Part model, mm, in its own coordinate system. A direction names the side the tool comes from. Give positions to 0.01 mm unless a question says otherwise; leave off trailing zeros. Order: outer loops, then holes, each group sorted by start corner. A loop starts at its lowest first (then second) coordinate and runs counter-clockwise, first axis right, second up. Notation, with made-up numbers: M -19.75,-22.75 L 13.25,-22.75 A23 ccw 13.25,-9.75 Z; hole C 24.25,48 d5. An arc over 180 degrees is marked long. Return JSON: item names as keys, results as strings.
Autodesk Inventor part; units mm, degrees
ref_plane "YZ Plane" through (0, 0, 0) normal (1, 0, 0) x (0, 1, 0)
ref_plane "XZ Plane" through (0, 0, 0) normal (0, 1, 0) x (-1, 0, 0)
ref_plane "XY Plane" through (0, 0, 0) normal (0, 0, 1) x (1, 0, 0)
sketch "Sketch1" plane through (0, 0, 0) normal (0, 1, 0) x (-1, 0, 0)
  line L0 (0, 0) -> (50.8, 0)
  line L1 (50.8, 0) -> (50.8, -9.525)
  line L2 (0, -9.525) -> (0, 0)
  line L3 (50.8, -9.525) -> (9.4322, -9.525)
  line L4 (3.3434, -9.525) -> (0, -9.525)
  arc A0 (9.4322, -9.525) -> (3.3434, -9.525) centre (6.3878, -11.9396) ccw
  point P0 (3.3434, 0)
  dimension "d1" = 9.525
revolve "Revolution1" add sketch "Sketch1" angle 360 about axis through (0, 0, 0) along (-1, 0, 0)
sketch "Sketch2" plane through (0, 0, 0) normal (1, 0, 0) x (0, 0, -1)
  circle A0 centre (0, 0) radius 3.81
  dimension "d3" = 7.62
extrude "Extrusion1" add sketch "Sketch2" along normal blind 1.5875
fillet "Fillet1" radius 1.27 2 edges at (0, 0, 9.525) (-50.8, 0, 9.525)
properties part number "bATTERY"
Q1. Probe line 1 along X through (y, z) = (-0.25, 7.5); line 2 along X through (y, z) = (-0.5, -8.5); line 3 along X through (y, z) = (-6, -6.25). List the from-to ranges inside material, lowest first.
Established:
{"line 1": "x = -50.8 to 0", "line 2": "x = -50.77 to -8.22, -4.55 to -0.03", "line 3": "x = -50.73 to -8.48, -4.3 to -0.07"}
Q2. 3-axis set-ups, long thin cutter, end or side, ignore diameter. For faces 1 (the flat face through (-50.8, 0, 0)), 2 (the flat face through (0, 2, -4)): which of +Z, -Z, +X, -X, +Y, -Y reach the whole face in a straight line?
Established:
{"face 1": "+Z, -Z, -X, +Y, -Y", "face 2": "+X"}
Q3. Pin check, flat tips, straight feed: pin 1 (6 mm diameter, centred on x = -34.5, z = -7.5, fed in from +Y) (3 decimals); pin 2 (5 mm diameter, centred on x = -39, y = 5.5, fed in from -Z). Stop position of each tip, or through.
Established:
{"pin 1": "stops at y = 8.395", "pin 2": "stops at z = -9.04"}
Q4. Band-saw the part on C-C (x = -45.5). Give the cut face in (y, z) (3 decimals), then the cut area to 3 significant figures.
Established:
{"outline": "C 0,0 d19.05", "area": "285 mm²"}
Q5. Band-saw the part on A-A (y = 0). Give the cut face in (x, z) (1 decimal), then the cut area to 3 significant figures.
Established:
{"outline": "M -50.8,-8.3 A1.3 ccw -49.5,-9.5 L -9.4,-9.5 A3.9 cw -3.3,-9.5 L -1.3,-9.5 A1.3 ccw 0,-8.3 L 0,-3.8 L 1.6,-3.8 L 1.6,3.8 L 0,3.8 L 0,8.3 A1.3 ccw -1.3,9.5 L -3.3,9.5 A3.9 cw -9.4,9.5 L -49.5,9.5 A1.3 ccw -50.8,8.3 Z", "area": "966 mm²"}
